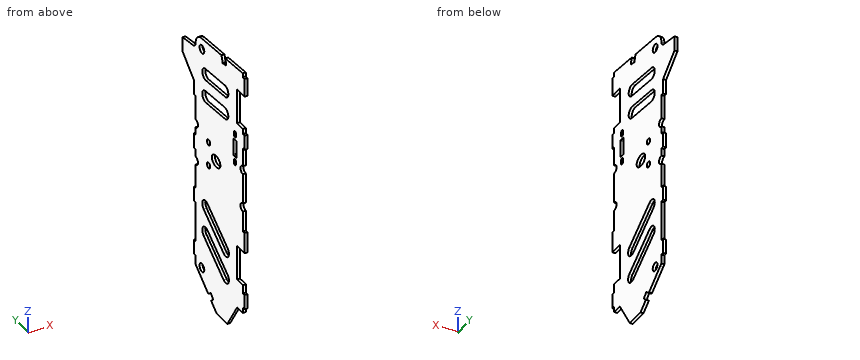
from build123d import *

# Parameters (mm, degrees)
SKETCH_218_R           = 2.25
EXTRUDE_1_DEPTH        = 1.6
SKETCH_2_W             = 8
SKETCH_2_H             = 1.6
EXTRUDE_3412_DEPTH     = 1.6
SKETCH2_W              = 19.07286805
SKETCH2_H              = 5.5
SKETCH2_H_2            = 5.238743847
SKETCH2_W_2            = 18.956012289
SKETCH2_H_3            = 4.1
CUT_EXTRUDE_4293_DEPTH = 113.482438083
SKETCH_4339_R          = 1.575
SKETCH_4339_RX         = 4.079397779
SKETCH_4339_RY         = 3.125
CUT_EXTRUDE_4732_DEPTH = 113.482438083
CUT_EXTRUDE_5198_DEPTH = 113.482438221
USB_C_DEPTH            = 113.482438221
BOSS_EXTRUDE1_DEPTH    = 1.6


with BuildPart() as part:
    # Sketch 218 → 凸台-拉伸1 (new body)
    with BuildSketch(Plane(origin=(0, 0, 0), x_dir=(0, 0, -1), z_dir=(1, 0, 0))):
        with BuildLine():
            Line((-95.193976275, 16.776432698), (-96.66172395, 0))
            Line((-96.66172395, 0), (-44.182229478, 0))
            ThreePointArc((-44.182229478, 0), (-41.932229478, 2.25), (-39.682229478, 0))
            Line((-39.682229478, 0), (-23.132229478, 0))
            ThreePointArc((-23.132229478, 0), (-20.882229478, 2.25), (-18.632229478, 0))
            Line((-18.632229478, 0), (38.58827605, 0))
            Line((38.58827605, 0), (38.58827605, 5.363667343))
            Line((38.58827605, 5.363667343), (53.613979238, 14.877821069))
            Line((53.613979238, 14.877821069), (53.613979238, 25.082386187))
            Line((53.613979238, 25.082386187), (49.47062371, 30.265958003))
            ThreePointArc((49.47062371, 30.265958003), (48.71615842, 29.206772475), (47.878069959, 28.212438733))
            Line((47.878069959, 28.212438733), (45.32875497, 30.545040291))
            ThreePointArc((45.32875497, 30.545040291), (46.329625978, 31.78976103), (47.163951689, 33.151735001))
            Line((47.163951689, 33.151735001), (38.58827605, 43.88038965))
            Line((38.58827605, 43.88038965), (37.693344157, 45))
            Line((37.693344157, 45), (-18.632229478, 45))
            ThreePointArc((-18.632229478, 45), (-20.882229478, 42.75), (-23.132229478, 45))
            Line((-23.132229478, 45), (-39.682229478, 45))
            ThreePointArc((-39.682229478, 45), (-41.932229478, 42.75), (-44.182229478, 45))
            Line((-44.182229478, 45), (-87.226747047, 45))
            ThreePointArc((-87.226747047, 45), (-91.280288293, 43.423664021), (-93.203915236, 39.522934456))
            Line((-93.203915236, 39.522934456), (-94.87665585, 20.403421746))
            ThreePointArc((-94.87665585, 20.403421746), (-92.972963578, 19.729950103), (-91.011324976, 19.250802615))
            Line((-91.011324976, 19.250802615), (-91.670050843, 15.813350036))
            ThreePointArc((-91.670050843, 15.813350036), (-93.450669808, 16.226628035), (-95.193976275, 16.776432698))
        make_face()
        with Locations((-87.226747047, 39)):
            Circle(SKETCH_218_R, mode=Mode.SUBTRACT)
        with Locations((36.08827605, 39)):
            Circle(SKETCH_218_R, mode=Mode.SUBTRACT)
    extrude(amount=EXTRUDE_1_DEPTH)

    # 草图2 → Extrude 3412 (add)
    with BuildSketch(Plane(origin=(0, 0, 0), x_dir=(0, 0, -1), z_dir=(1, 0, 0))):
        with Locations((31.58827605, -0.8)):
            Rectangle(SKETCH_2_W, SKETCH_2_H)
        with BuildLine():
            Line((-83.150237988, 57.5), (-84.607683433, 47.272305319))
            ThreePointArc((-84.607683433, 47.272305319), (-85.493046837, 45.647255317), (-87.226747047, 45))
            Line((-87.226747047, 45), (-65.306655843, 45))
            Line((-65.306655843, 45), (-57.306655843, 45))
            Line((-57.306655843, 45), (-57.306655843, 46.6))
            Line((-57.306655843, 46.6), (-65.306655843, 46.6))
            Line((-65.306655843, 46.6), (-75.139107316, 57.5))
            Line((-75.139107316, 57.5), (-83.150237988, 57.5))
        make_face()
        with Locations((1.58827605, -0.8)):
            Rectangle(SKETCH_2_W, SKETCH_2_H)
        with Locations((-58.41172395, -0.8)):
            Rectangle(SKETCH_2_W, SKETCH_2_H)
        with Locations((-88.41172395, -0.8)):
            Rectangle(SKETCH_2_W, SKETCH_2_H)
        with Locations((28.693344157, 45.8)):
            Rectangle(SKETCH_2_W, SKETCH_2_H)
        with Locations((-1.306655843, 45.8)):
            Rectangle(SKETCH_2_W, SKETCH_2_H)
        with Locations((-31.306655843, 45.8)):
            Rectangle(SKETCH_2_W, SKETCH_2_H)
    extrude(amount=EXTRUDE_3412_DEPTH)

    # Sketch2 → Cut-Extrude 4293 (cut, through all)
    with BuildSketch(Plane(origin=(1.6, 0, 0), x_dir=(0, 0, -1), z_dir=(1, 0, 0))):
        with Locations((-74.777688237, 2.75)):
            Rectangle(SKETCH2_W, SKETCH2_H)
        with Locations((-74.777688237, -2.619371924)):
            Rectangle(SKETCH2_W, SKETCH2_H_2)
        with Locations((13.467678305, 2.75)):
            Rectangle(SKETCH2_W_2, SKETCH2_H)
        with Locations((13.467678305, -2.05)):
            Rectangle(SKETCH2_W_2, SKETCH2_H_3)
    extrude(amount=-CUT_EXTRUDE_4293_DEPTH, mode=Mode.SUBTRACT)

    # Sketch 4339 → Cut-Extrude 4732 (cut, through all)
    with BuildSketch(Plane(origin=(1.6, 0, 0), x_dir=(0, 0, -1), z_dir=(1, 0, 0))):
        with Locations((-38.41172395, 32.651369249)):
            Circle(SKETCH_4339_R)
        with Locations((-25.41172395, 32.651369249)):
            Circle(SKETCH_4339_R)
        with Locations(Location((-31.91172395, 25.5), (0, 0, 90))):
            Ellipse(SKETCH_4339_RX, SKETCH_4339_RY)
    extrude(amount=-CUT_EXTRUDE_4732_DEPTH, mode=Mode.SUBTRACT)

    # 草图3 → Cut-Extrude 5198 (cut, through all)
    with BuildSketch(Plane(origin=(1.6, 0, 0), x_dir=(0, 0, -1), z_dir=(1, 0, 0))):
        with BuildLine():
            Line((-71.837081834, 35.223280517), (-73.455622109, 16.723280517))
            ThreePointArc((-73.455622109, 16.723280517), (-76.895259758, 13.837081834), (-79.781458442, 17.276719483))
            Line((-79.781458442, 17.276719483), (-78.162918166, 35.776719483))
            ThreePointArc((-78.162918166, 35.776719483), (-74.723280517, 38.662918166), (-71.837081834, 35.223280517))
        make_face()
        with BuildLine():
            Line((17.026747393, 37.354992688), (30.756614535, 18.283004112))
            ThreePointArc((30.756614535, 18.283004112), (30.034859831, 13.851264031), (25.60311975, 14.573018735))
            Line((25.60311975, 14.573018735), (11.873252607, 33.645007312))
            ThreePointArc((11.873252607, 33.645007312), (12.595007312, 38.076747393), (17.026747393, 37.354992688))
        make_face()
        with BuildLine():
            Line((2.026747393, 37.354992688), (15.756614535, 18.283004112))
            ThreePointArc((15.756614535, 18.283004112), (15.034859831, 13.851264031), (10.60311975, 14.573018735))
            Line((10.60311975, 14.573018735), (-3.126747393, 33.645007312))
            ThreePointArc((-3.126747393, 33.645007312), (-2.404992688, 38.076747393), (2.026747393, 37.354992688))
        make_face()
        with BuildLine():
            Line((-59.337081834, 35.223280517), (-60.955622109, 16.723280517))
            ThreePointArc((-60.955622109, 16.723280517), (-64.395259758, 13.837081834), (-67.281458442, 17.276719483))
            Line((-67.281458442, 17.276719483), (-65.662918166, 35.776719483))
            ThreePointArc((-65.662918166, 35.776719483), (-62.223280517, 38.662918166), (-59.337081834, 35.223280517))
        make_face()
    extrude(amount=-CUT_EXTRUDE_5198_DEPTH, mode=Mode.SUBTRACT)

    # Sketch1 → USB-C供电接口 (cut, through all)
    with BuildSketch(Plane(origin=(0, 0, 0), x_dir=(0, 0, -1), z_dir=(1, 0, 0))):
        with BuildLine():
            Line((-54.375, 9), (-45.625, 9))
            ThreePointArc((-45.625, 9), (-45.271446609, 8.853553391), (-45.125, 8.5))
            Line((-45.125, 8.5), (-45.125, 6.5))
            ThreePointArc((-45.125, 6.5), (-45.271446609, 6.146446609), (-45.625, 6))
            Line((-45.625, 6), (-54.375, 6))
            ThreePointArc((-54.375, 6), (-54.728553391, 6.146446609), (-54.875, 6.5))
            Line((-54.875, 6.5), (-54.875, 8.5))
            ThreePointArc((-54.875, 8.5), (-54.728553391, 8.853553391), (-54.375, 9))
        make_face()
        with BuildLine():
            Line((-57.25, 6.475), (-58.5, 6.475))
            ThreePointArc((-58.5, 6.475), (-59.525, 7.5), (-58.5, 8.525))
            Line((-58.5, 8.525), (-57.25, 8.525))
            ThreePointArc((-57.25, 8.525), (-56.225, 7.5), (-57.25, 6.475))
        make_face()
        with BuildLine():
            Line((-42.75, 6.475), (-41.5, 6.475))
            ThreePointArc((-41.5, 6.475), (-40.475, 7.5), (-41.5, 8.525))
            Line((-41.5, 8.525), (-42.75, 8.525))
            ThreePointArc((-42.75, 8.525), (-43.775, 7.5), (-42.75, 6.475))
        make_face()
    extrude(amount=USB_C_DEPTH, mode=Mode.SUBTRACT)

    # Sketch3 → Boss-Extrude1 (add)
    with BuildSketch(Plane(origin=(1.6, 0, 0), x_dir=(0, 0, -1), z_dir=(1, 0, 0))):
        Polygon((-92.41172395, -1.6), (-94.41172395, -1.6), (-94.41172395, 0), (-94.41172395, 0.25), (-92.16172395, 0.25), (-92.16172395, -1.6), align=None)
        Polygon((-2.41172395, -1.6), (-7.41172395, -1.6), (-7.41172395, 0), (-7.41172395, 0.25), (-2.16172395, 0.25), (-2.16172395, -1.6), align=None)
    extrude(amount=-BOSS_EXTRUDE1_DEPTH)


solid = part.part
Verification items for the finished model (mm, model axes). Coordinates: 2 decimals unless noted, no trailing zeros. Loops run counter-clockwise (first coordinate to the right, second up) from the corner with the lowest first, then second, coordinate; pieces in that order, holes last. Notation, with made-up numbers: (78.25, -5.5) -> (126.25, -5.5) arc R16 cw to (126.25, -0.5) -> close; hole circle Ø7 at (-7.75, 66.25). An arc over 180 degrees is marked (long way). Answer as CSV lines item,"result".
1) Cross-section at C-C, the plane y = 10.5. Record the cut outline in (x, z).
Found:
outline,"(0, -46.7) -> (1.6, -46.7) -> (1.6, 95.74) -> (0, 95.74) -> close"
2) Depth check by flat-ended pin: pin 1 (0.8 mm diameter, centred on x = 0.5, z = 10.5, fed in from -Y); pin 2 (0.8 mm diameter, centred on x = 1, y = 4, fed in from +Z); pin 3 (0.5 mm diameter, centred on x = 1, y = -1, fed in from +Z). Enter the tip coordinate at first touch or a pass-through.
Found:
pin 1,"stops at y = 0"
pin 2,"stops at z = 96.35"
pin 3,"stops at z = 94.41"
3) Cross-section at A-A, the plane z = 0.55. Record the cut outline in (x, y) (3 decimals).
Found:
outline,"(0, -1.6) -> (1.6, -1.6) -> (1.6, 30.066) -> (0, 30.066) -> close; (0, 38.675) -> (1.6, 38.675) -> (1.6, 46.6) -> (0, 46.6) -> close"
4) Cross-section at B-B, the plane x = 1.05. Count the separate pieces of the cut face and the enclosed holes in it, then the cut area to 3 significant figures.
Found:
separate pieces,"1"
enclosed holes,"12"
area,"5,600 mm2"
5) Thickness scan on L1, parallel to Y at x = 0.1, z = 57.5 (3 decimals); L2, parallel to Z at x = 1.55, y = 13.5; L3, parallel to Z at x = 1.4, y = 4.5. Record the ranges inside material, lowest first. Write a range as from..to.
Found:
L1,"y = -1.6..6.475, 8.525..46.6"
L2,"z = -51.44..-29.41, -26.95..-14.41, -11.95..95.48"
L3,"z = -38.59..-22.95, -3.99..65.24, 84.31..96.27"
